Here's how the part is built. I have some questions about the finished solid (model axes, mm). A direction names the side the tool comes from. Coordinates: 2 decimals unless noted, no trailing zeros. Write each loop counter-clockwise with the first axis right and the second up, starting at its lowest first coordinate (ties: lowest second). Pieces come first, ordered by that corner, then holes.
Item 1: If we section it at A-A (x = 0): Please give me the cut outline in (y, z).
Item 2: We'd pull the mould along X, two halves only. Please class faces 1 (the face through (-1, 0, 18)), 2 (the face through (13.858, 15.653, -10.626)), 3 (the face through (0, 0, 0)): +X half, -X half, draft (parallel to the pull), parting line (faces both ways), or undercut.
Item 3: I'm going to push flat-ended pins straight in: pin 1 Ø8 at (x, z) = (43.5, 3) entering from -Y; pin 2 Ø12 at (y, z) = (4.5, -60) entering from +X; pin 3 Ø6 at (x, z) = (-9, 52) entering from +Y. Where does each tip first touch, or does it pass through?
Item 4: For faces 4 (the face through (-10.6, 15.65, 3.34)), 5 (the face through (-2.44, -24.17, -10.98)), which set-ups out of +Z, -Z, +X, -X, +Y, -Y let a thin tool reach every point of the face, with its end or its side?
Item 5: If we section it at B-B (y = 19.5): Please give me the cut outline in (x, z) (1 decimal), then the cut area to 3 significant figures.
Item 6: If we section it at D-D (y = -21): Please give me the cut outline in (x, z) (1 decimal), then the cut area to 3 significant figures.
Item 7: If I drill on line 1 (Z direction, x = 0, y = 17); line 2 (X direction, y = 15.5, z = 7); line 3 (Y direction, x = -55.5, z = -12.5), over which ranges is the centre line in solid material (lowest first)?
Item 8: If we section it at C-C (y = -2.5): Please give me the cut outline in (x, z).
from build123d import *

# Parameters (mm, degrees)
F0_R     = 76.2
F2_R     = 7.9375
F4_R     = 17.4625
F4_R_2   = 11.1125
F5_DEPTH = 31.75


with BuildPart() as f3:
    # F0 (on Front) → F3 section 0
    with BuildSketch(Plane.XZ):
        Circle(F0_R)
    # F2 (on offset) → F3 section 1
    with BuildSketch(Plane.XZ.offset(25.4)):
        Circle(F2_R)
    loft()

    # F4 (on face) → F5 (join)
    with BuildSketch(Plane(origin=(0, 0, 0), x_dir=(-1, 0, 0), z_dir=(0, 1, 0))):
        Circle(F4_R)
        Circle(F4_R_2, mode=Mode.SUBTRACT)
    extrude(amount=F5_DEPTH)


solid = f3.part
Answer list:
1. outline: (-25.4, -7.94) - (0, -76.2) - (0, -17.46) - (31.75, -17.46) - (31.75, -11.11) - (0, -11.11) - (0, 11.11) - (31.75, 11.11) - (31.75, 17.46) - (0, 17.46) - (0, 76.2) - (-25.4, 7.94) - close
2. face 1: draft
2. face 2: parting line
2. face 3: undercut
3. pin 1: stops at y = -13.62
3. pin 2: stops at x = 51.64
3. pin 3: stops at y = 0
4. face 4: +Y
4. face 5: -Y
5. outline: circle Ø34.9 at (0, 0); hole circle Ø22.2 at (0, 0)
5. area: 570 mm2
6. outline: circle Ø39.5 at (0, 0)
6. area: 1,230 mm2
7. line 1: z = -17.46 to -11.11, 11.11 to 17.46
7. line 2: x = -16 to -8.63, 8.63 to 16
7. line 3: y = -7.19 to 0
8. outline: circle Ø138.96 at (0, 0)
